from build123d import *

# Parameters (mm, degrees)
BOSS_EXTRUDE1_DEPTH                         = 3.175
SKETCH2_R                                   = 6.35
BOSS_EXTRUDE2_DEPTH                         = 25.4
CSK_START                                   = -3
CSK_FOR_4_FLAT_HEAD_MACHINE_SCREW_2_R       = 1.63195
CSK_FOR_4_FLAT_HEAD_MACHINE_SCREW_100_DEPTH = 3.290441965
FILLET1_R                                   = 5


with BuildPart() as part:
    # Sketch3 → Boss-Extrude1 (new body)
    with BuildSketch(Plane(origin=(0, 0, 0), x_dir=(1, 0, 0), z_dir=(0, 1, 0))):
        with BuildLine():
            Line((-14.617805765, 29.891737943), (27.723314788, -12.932962722))
            Line((27.723314788, -12.932962722), (0, -12.869393963))
            ThreePointArc((0, -12.869393963), (-10.348328742, -9.868233169), (-14.787821417, -0.050607252))
            Line((-14.787821417, -0.050607252), (-14.617805765, 29.891737943))
        make_face()
        with BuildLine():
            Line((15.324539429, 29.721722291), (-14.617805765, 29.891737943))
            Line((-14.617805765, 29.891737943), (27.723314788, -12.932962722))
            Line((27.723314788, -12.932962722), (27.974571526, 14.789286355))
            ThreePointArc((27.974571526, 14.789286355), (25.091118162, 25.171028529), (15.324539429, 29.721722291))
        make_face()
    extrude(amount=BOSS_EXTRUDE1_DEPTH)

    # Sketch2 → Boss-Extrude2 (add)
    with BuildSketch(Plane(origin=(0, 0, 0), x_dir=(1, 0, 0), z_dir=(0, 1, 0))):
        with BuildLine():
            Line((2.835804927, -0.290441965), (10.269704096, -0.290441965))
            ThreePointArc((10.269704096, -0.290441965), (16.077754512, 8.47938761), (10.269704096, 17.249217186))
            Line((10.269704096, 17.249217186), (2.835804927, 17.249217186))
            ThreePointArc((2.835804927, 17.249217186), (-2.972245488, 8.47938761), (2.835804927, -0.290441965))
        make_face()
        with Locations(Location((6.552754512, 8.47938761, 0), (0, 0, 270))):
            Circle(SKETCH2_R, mode=Mode.SUBTRACT)
    extrude(amount=-BOSS_EXTRUDE2_DEPTH)

    # CSK for #4 Flat Head Machine Screw (100)1: read off the stored shape, not the designer's step
    # CSK for _4 Flat Head Machine Screw _ 2 → CSK for #4 Flat Head Machine Screw (100)1 (cut)
    with BuildSketch(Plane.XY.offset(CSK_START)):
        with Locations((6.81485322, -12.7)):
            Circle(CSK_FOR_4_FLAT_HEAD_MACHINE_SCREW_2_R)
    extrude(amount=CSK_FOR_4_FLAT_HEAD_MACHINE_SCREW_100_DEPTH, mode=Mode.SUBTRACT)

    # CSK for _4 Flat Head Machine Screw _ 3 o → CSK for _4 Flat Head Machine Screw _ 3 (revolve, cut)
    with BuildSketch(Plane(origin=(6.81485322, -12.7, 0), x_dir=(1, 0, 0), z_dir=(0, -1, 0))):
        Polygon((1.63195, 0.290441965), (1.63195, -0.737916588), (2.8575, 0.290441965), align=None)
    revolve(axis=Axis((6.81485322, -12.7, 0), (0, 0, 1)), mode=Mode.SUBTRACT)

    # Fillet1
    fillet1_edges = [part.edges().sort_by_distance(p)[0] for p in [
        (-2.972245488, 0, -8.47938761),
        (16.077754512, 0, -8.47938761),
    ]]
    fillet(fillet1_edges, radius=FILLET1_R)


solid = part.part
Work out the finished part from the listing and answer in its coordinate system (mm). A direction names the side the tool comes from. Round coordinates to 2 decimals unless told otherwise and drop trailing zeros. Write each loop counter-clockwise with the first axis right and the second up, starting at its lowest first coordinate (ties: lowest second). Pieces come first, ordered by that corner, then holes. Notation, with made-up numbers: (-17.75, 14) - (28.25, 14) arc R21 cw to (28.25, 18) - close; hole circle Ø11 at (30, 42.5). An arc over 180 degrees is marked (long way). Answer in a Markdown table with one row per item. Add a question column.
1. A cutting plane is placed at B-B, the plane y = -12.7. Determine the outline of the cut face in (x, z) (3 decimals), and give its area (3 significant figures).
2. Given pin 1 (8 mm diameter, centred on x = 4, y = -13.5, fed in from -Z); pin 2 (2 mm diameter, centred on y = -20, z = -7.5, fed in from +X); pin 3 (4 mm diameter, centred on x = 5, z = -7, fed in from -Y), each flat-ended and moving along its own axis, determine where each tip first touches the part or whether it passes through.
3. A cutting plane is placed at C-C, the plane z = -23.5. Determine the outline of the cut face in (x, y) (3 decimals).
4. For faces 1 (the flat face through (5, -10, 0.29)), 2 (the flat face through (7, -14, -17.249)), 3 (the flat face through (7, 0, -9)), determine the directions among +Z, -Z, +X, -X, +Y, -Y from which every point of the face is accessible in a straight line to the end or side of a thin tool.
5. A cutting plane is placed at D-D, the plane x = 25.5. Determine the outline of the cut face in (y, z) (3 decimals).
6. The mould has two halves that part along X. Classify faces 4 (the cylindrical face through (11.91, -12.52, -5.07)), 5 (the cylindrical face through (8.37, -12.21, -1.59)), 6 (the cylindrical face through (16.076, -15.057, -8.323)), 7 (the flat face through (7, 0, 1)): +X half, -X half, draft (parallel to the pull), parting line (faces both ways), or undercut.
7. A cutting plane is placed at A-A, the plane y = -7.5. Determine the outline of the cut face in (x, z) (3 decimals), and give its area (3 significant figures).
8. Find the intervals of material crossed by line 1 along Y through (x, z) = (12, 11) (3 decimals); line 2 along Z through (x, y) = (2.5, -7.75); line 3 along X through (y, z) = (-12.7, -1.95), in increasing order. Write a range as from..to.
Worked out:
| question | item | result |
|---|---|---|
| 1 | outline | (2.836, -17.249) - (10.27, -17.249) arc R9.525 ccw to (10.27, 0.29) - (9.672, 0.29) - (8.447, -0.738) - (8.447, -2.418) arc R6.35 cw (long way) to (5.183, -2.279) - (5.183, -0.738) - (3.957, 0.29) - (2.836, 0.29) arc R9.525 ccw to start |
| 1 | area | 141 mm^2 |
| 2 | pin 1 | z = -17.25 |
| 2 | pin 2 | x = 16.08 |
| 2 | pin 3 | y = 0 |
| 3 | outline | (-14.654, 0) - (26.291, 0) - (26.291, 3.175) - (-14.654, 3.175) - close |
| 4 | face 1 | +Z, +X, -X, -Y |
| 4 | face 2 | -Z, +X, -X, -Y |
| 4 | face 3 | -Y |
| 5 | outline | (0, -24.663) - (3.175, -24.663) - (3.175, 12.928) - (0, 12.928) - close |
| 6 | face 4 | undercut |
| 6 | face 5 | undercut |
| 6 | face 6 | +X half |
| 6 | face 7 | draft |
| 7 | outline | (2.836, -17.249) - (10.27, -17.249) arc R9.525 ccw to (10.27, 0.29) - (2.836, 0.29) arc R9.525 ccw to start; hole circle Ø12.7 at (6.553, -8.479) |
| 7 | area | 151 mm^2 |
| 8 | line 1 | 0..3.175 |
| 8 | line 2 | -17.1..-13.37, -3.59..0.14 |
| 8 | line 3 | -0.38..5.18, 8.45..13.49 |
